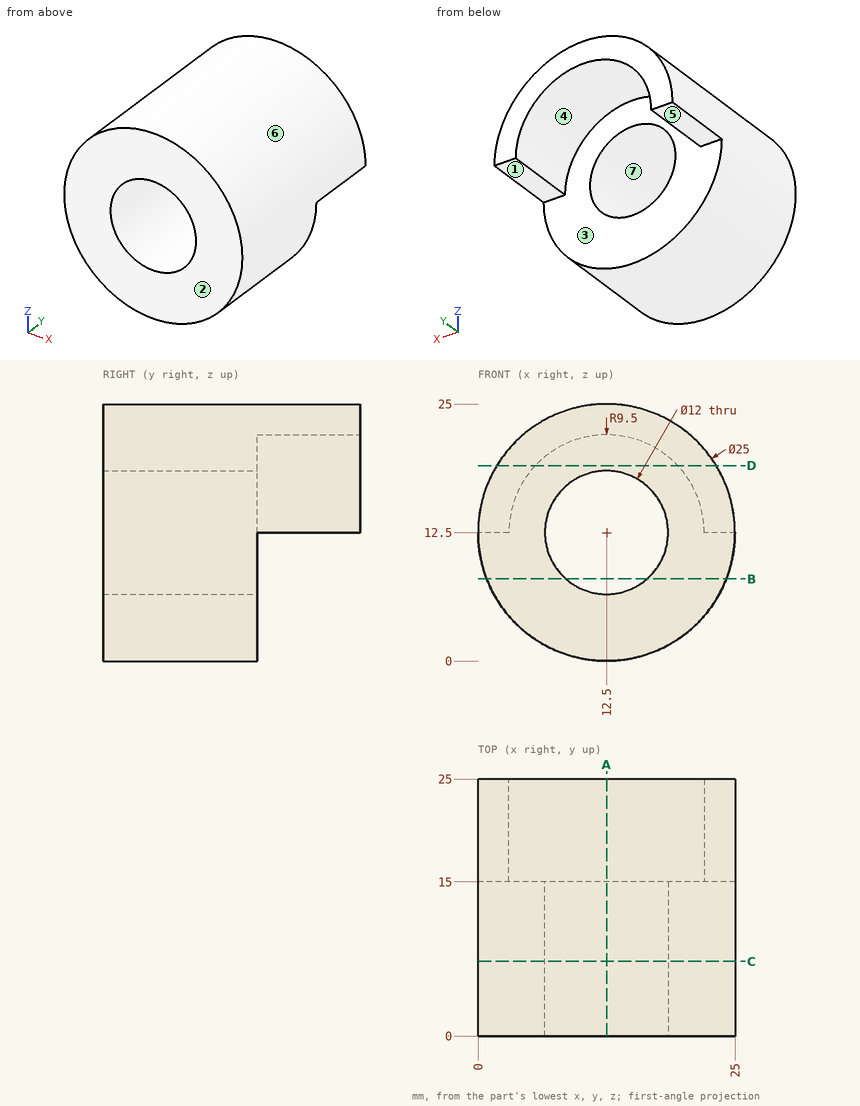
Could you check a few things on this drawing? It's one solid part, dimensions in mm from its lowest x, y, z. A direction names the side the tool comes from. Round coordinates to 2 decimals unless told otherwise and drop trailing zeros. Write each loop counter-clockwise with the first axis right and the second up, starting at its lowest first coordinate (ties: lowest second). Pieces come first, ordered by that corner, then holes. Notation, with made-up numbers: (84, 7) -> (95, 7) arc R18 ccw to (95, 13) -> close; hole circle Ø2 at (44, -26.5). An arc over 180 degrees is marked (long way). One line per question, with ' | ' between items. Start each with the question number.
1) Suppose I cut it at C-C on y = 7.25. Write out the boundary of the cut face in (x, z).
2) On a 3-axis mill with a long thin cutter (end or side, diameter ignored), from which of +Z, -Z, +X, -X, +Y, -Y can I reach the whole of each face in a straight line? I mean the marked faces 1, 2 and 3. Say none if no direction works.
3) Suppose I cut it at D-D on z = 19. Write out the boundary of the cut face in (x, y), then the cut area to 3 significant figures.
4) I'm going to push flat-ended pins straight in: P1, Ø6, axis at y = 3, z = 20.5, coming from the +X side; P2, Ø1.5, axis at x = 9.5, z = 19.5, coming from the +Y side; P3, Ø10, axis at y = 13, z = 4, coming from the +X side. Where does each tip first touch, or does it pass through?
5) Suppose I cut it at A-A on x = 12.5. Write out the boundary of the cut face in (y, z), then the cut area to 3 significant figures.
6) I need wall thicknesses on line 1 (Z direction, x = 12.5, y = 5); line 2 (Y direction, x = 4.25, z = 9); line 3 (X direction, y = 21.5, z = 16.75). Which ranges of each line are inside material? Lowest first, please. Write a range as [from, to].
7) If we mould it in two halves opening along X, with no side actions, what happens to the marked faces 4, 5, 6 and 7? For each: released by +X, released by -X, zero draft, split by the parting line, or undercut.
8) Suppose I cut it at B-B on z = 8. Write out the boundary of the cut face in (x, y).
Return value:
1) outline: circle Ø25 at (12.5, 12.5); hole circle Ø12 at (12.5, 12.5)
2) face 1: -Z, +X, -X, +Y | face 2: +Z, -Z, +X, -X, -Y | face 3: -Z, +Y
3) outline: (1.82, 0) -> (23.18, 0) -> (23.18, 25) -> (19.43, 25) -> (19.43, 15) -> (5.57, 15) -> (5.57, 25) -> (1.82, 25) -> close | area: 395 mm2
4) P1: stops at x = 23.96 | P2: stops at y = 15 | P3: stops at x = 24.5
5) outline: (0, 0) -> (15, 0) -> (15, 6.5) -> (0, 6.5) -> close; (0, 18.5) -> (15, 18.5) -> (15, 22) -> (25, 22) -> (25, 25) -> (0, 25) -> close | area: 225 mm2
6) line 1: z = [0, 6.5], [18.5, 25] | line 2: y = [0, 15] | line 3: x = [0.74, 4], [21, 24.26]
7) face 4: undercut | face 5: zero draft | face 6: split by the parting line | face 7: undercut
8) outline: (0.84, 0) -> (8.53, 0) -> (8.53, 15) -> (0.84, 15) -> close; (16.47, 0) -> (24.16, 0) -> (24.16, 15) -> (16.47, 15) -> close
